Design review of the part built by this model. Coordinates are the model's own, in mm. Coordinates: 2 decimals unless noted, no trailing zeros. Loops run counter-clockwise (first coordinate to the right, second up) from the corner with the lowest first, then second, coordinate; pieces in that order, holes last. Notation, with made-up numbers: M 71,29 L 128,29 A14 cw 128,41 Z; hole C 14,9 d7. An arc over 180 degrees is marked long. Put each result on its own line as item: value. Start each with the question number.
(1) The part is to be moulded in two halves that separate along X. For faces 1 (the flat face through (-1.875, -1.1, -1.3)), 2 (the cylindrical face through (-1.51, -5.37, -1.19)), 3 (the flat face through (-0.375, 0.5, -1.6)), 4 (the cylindrical face through (-0.005, -4.214, 2.192)), say which applies: +X half, -X half, draft (parallel to the pull), parting line (faces both ways), or undercut.
(2) For probe 1 along Y at (x, z) = (-0.3, -0.5); probe 2 along Z at (x, y) = (-0.8, 0) (3 decimals); probe 3 along Z at (x, y) = (-1.05, 0) (3 decimals), list the stretches that pass through material, from the lowest coordinate up. Write a range as [from, to].
(3) Take a section at A-A, the plane x = -1.6. Give the boundary of the cut face in (y, z), then the cut area to 3 significant figures.
```python
from build123d import *

# Parameters (mm, degrees)
F2_R     = 1.5
F3_DEPTH = 2.25
F4_DEPTH = 3.751


with BuildPart() as f1:
    # F0 (on Front) → F1 (revolve)
    with BuildSketch(Plane.XZ):
        Polygon((-1.875, 5.5), (-1.875, 0), (1.875, 0), (1.875, 5.5), (1.125, 5.5), (0.375, 4.75), (-0.375, 4.75), (-1.125, 5.5), align=None)
    revolve(axis=Axis((0, 0, 0), (-1, 0, 0)))

    # F2 (on face) → F3 (cut)
    with BuildSketch(Plane.YZ.offset(1.875)):
        Polygon((-0.6335184836, 1.9496536007), (-1.0462478749, 2.1599497294), (-1.1325303049, 2.1159866355), (-1.2049934123, 1.6584725808), (-1.662507467, 1.7309356883), (-1.7309815911, 1.6624615642), (-1.6585184836, 1.2049475095), (-2.1160325383, 1.132484402), (-2.1599956322, 1.0462019721), (-1.9496995035, 0.6334725808), (-2.3624288949, 0.4231764522), (-2.3775775446, 0.3275316418), (-2.0500336451, -1.22577e-05), (-2.3775775446, -0.3275561571), (-2.3624288949, -0.4232009675), (-1.9496995035, -0.6334970961), (-2.1599956322, -1.0462264874), (-2.1160325383, -1.1325089174), (-1.6585184836, -1.2049720249), (-1.7309815911, -1.6624860795), (-1.662507467, -1.7309602036), (-1.2049934123, -1.6584970961), (-1.1325303049, -2.1160111508), (-1.0462478749, -2.1599742447), (-0.6335184836, -1.9496781161), (-0.423222355, -2.3624075074), (-0.3275775446, -2.3775561571), (-3.36451e-05, -2.0500122577), (0.3275102543, -2.3775561571), (0.4231550647, -2.3624075074), (0.6334511933, -1.9496781161), (1.0461805846, -2.1599742447), (1.1324630146, -2.1160111508), (1.2049261221, -1.6584970961), (1.6624401767, -1.7309602036), (1.7309143008, -1.6624860795), (1.6584511933, -1.2049720249), (2.115965248, -1.1325089174), (2.1599283419, -1.0462264874), (1.9496322133, -0.6334970961), (2.3623616046, -0.4232009675), (2.3775102543, -0.3275561571), (2.0499663549, -1.22577e-05), (2.3775102543, 0.3275316418), (2.3623616046, 0.4231764522), (1.9496322133, 0.6334725808), (2.1599283419, 1.0462019721), (2.115965248, 1.132484402), (1.6584511933, 1.2049475095), (1.7309143008, 1.6624615642), (1.6624401767, 1.7309356883), (1.2049261221, 1.6584725808), (1.1324630146, 2.1159866355), (1.0461805846, 2.1599497294), (0.6334511933, 1.9496536007), (0.4231550647, 2.3623829921), (0.3275102543, 2.3775316418), (-3.36451e-05, 2.0499877423), (-0.3275775446, 2.3775316418), (-0.423222355, 2.3623829921), align=None)
        Circle(F2_R, mode=Mode.SUBTRACT)
    extrude(amount=-F3_DEPTH, mode=Mode.SUBTRACT)

    # F2 (on face) → F4 (cut, through all)
    with BuildSketch(Plane.YZ.offset(1.875)):
        Circle(F2_R)
    extrude(amount=-F4_DEPTH, mode=Mode.SUBTRACT)


solid = f1.part
```
Computed values:
1. face 1: -X half
1. face 2: draft
1. face 3: +X half
1. face 4: undercut
2. probe 1: y = [-4.72, -2.21], [2.21, 4.72]
2. probe 2: z = [-5.175, -1.5], [1.5, 5.175]
2. probe 3: z = [-5.425, -1.5], [1.5, 5.425]
3. outline: C 0,0 d11; hole C 0,0 d3
3. area: 88.0 mm^2
